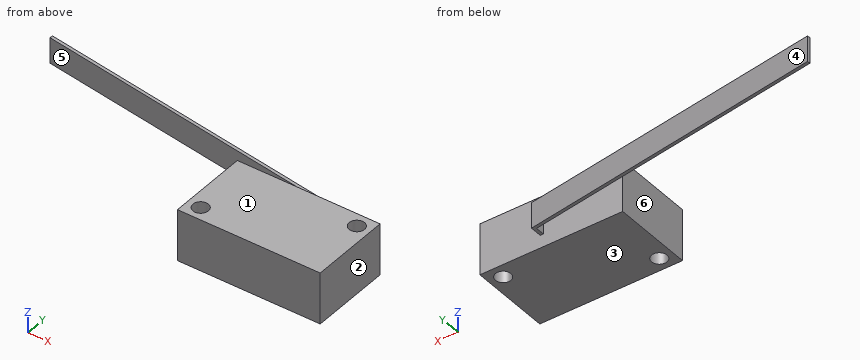
from build123d import *

# Parameters (mm, degrees)
SKETCH_1_W        = 27.7
SKETCH_1_H        = 15.8
SKETCH_1_R        = 1.5
EXTRUDE_1_DEPTH   = 5
EXTRUDE_1_2_DEPTH = 2.5


with BuildPart() as part:
    # ｽｹｯﾁ1 → Extrude 1 (new, symmetric)
    with BuildSketch(Plane.XY):
        Rectangle(SKETCH_1_W, SKETCH_1_H)
        with Locations((11.25, 5.3)):
            Circle(SKETCH_1_R, mode=Mode.SUBTRACT)
        with Locations((-11.25, -5.3)):
            Circle(SKETCH_1_R, mode=Mode.SUBTRACT)
    extrude(amount=EXTRUDE_1_DEPTH, both=True)

    # ｽｹｯﾁ2 → Extrude 1 2 (add, symmetric)
    with BuildSketch(Plane.XY):
        Polygon((2.15, 7.9), (2.15, 10.2), (-58.15, 19.414662229), (-58.240636022, 18.821547475), (1.55, 9.684723007), (1.55, 7.9), align=None)
    extrude(amount=EXTRUDE_1_2_DEPTH, both=True)


solid = part.part
Work out the finished part from the listing and answer in its coordinate system (mm). Face numbers are marked on the shaded views. A direction names the side the tool comes from. Coordinates: 2 decimals unless noted, no trailing zeros. Write each loop counter-clockwise with the first axis right and the second up, starting at its lowest first coordinate (ties: lowest second). Pieces come first, ordered by that corner, then holes.
1. For a pull along Z with two mould halves and no side action, classify the marked faces 1, 2 and 3 as +Z half, -Z half, draft (parallel to the pull), parting line (faces both ways), or undercut.
Results list:
face 1: +Z half
face 2: draft
face 3: -Z half
2. Consider line 1 along X through (y, z) = (5.25, -3.5); line 2 along Y through (x, z) = (11.25, -2.25); line 3 along X through (y, z) = (8, 1.5). Determine where each line is inside the solid, lowest interval first.
Results list:
line 1: x = -13.85 to 9.75, 12.75 to 13.85
line 2: y = -7.9 to 3.8, 6.8 to 7.9
line 3: x = 1.55 to 2.15
3. The part is cut by section C-C, the plane z = -1.75. Write down the section's boundary in (x, y).
Results list:
outline: (-58.24, 18.82) - (1.55, 9.68) - (1.55, 7.9) - (-13.85, 7.9) - (-13.85, -7.9) - (13.85, -7.9) - (13.85, 7.9) - (2.15, 7.9) - (2.15, 10.2) - (-58.15, 19.41) - close; hole circle Ø3 at (-11.25, -5.3); hole circle Ø3 at (11.25, 5.3)
4. For the marked faces 4, 5 and 6, determine the directions among +Z, -Z, +X, -X, +Y, -Y from which every point of the face is accessible in a straight line to the end or side of a thin tool.
Results list:
face 4: +Z, -Z, +X, +Y
face 5: +Z, -Z, -X
face 6: +Z, -Z, -X, -Y
5. Flat-ended cylindrical pins translate along their axes: pin 1 (12.5 mm diameter, centred on x = -27, y = 15.5, fed in from -Z); pin 2 (5 mm diameter, centred on x = 2, z = -2, fed in from +Y); pin 3 (4 mm diameter, centred on y = -2.5, z = -4, fed in from -X); pin 4 (2.5 mm diameter, centred on x = -11.25, y = -5.3, fed in from -Z). Find the tip coordinate at first contact, or state that the pin passes through.
Results list:
pin 1: stops at z = -2.5
pin 2: stops at y = 10.6
pin 3: stops at x = -13.85
pin 4: passes through
6. The part is cut by section B-B, the plane x = 11.25. Write down the section's boundary in (y, z).
Results list:
outline: (-7.9, -5) - (3.8, -5) - (3.8, 5) - (-7.9, 5) - close; (6.8, -5) - (7.9, -5) - (7.9, 5) - (6.8, 5) - close
7. The part is cut by section A-A, the plane y = -5.3. Write down the section's boundary in (x, z).
Results list:
outline: (-13.85, -5) - (-12.75, -5) - (-12.75, 5) - (-13.85, 5) - close; (-9.75, -5) - (13.85, -5) - (13.85, 5) - (-9.75, 5) - close
8. The part is cut by section D-D, the plane x = -11.25. Write down the section's boundary in (y, z).
Results list:
outline: (-7.9, -5) - (-6.8, -5) - (-6.8, 5) - (-7.9, 5) - close; (-3.8, -5) - (7.9, -5) - (7.9, 5) - (-3.8, 5) - close; (11.64, -2.5) - (12.25, -2.5) - (12.25, 2.5) - (11.64, 2.5) - close
